from build123d import *

# Parameters (mm, degrees)
SKETCH2_R           = 6
BOSS_EXTRUDE1_DEPTH = 15
SKETCH3_R           = 6
CUT_EXTRUDE1_DEPTH  = 27
SKETCH4_R           = 6
CUT_EXTRUDE2_DEPTH  = 27


with BuildPart() as part:
    # Sketch2 → Boss-Extrude1 (new body)
    with BuildSketch(Plane.XY):
        Polygon((0, 20.4), (5, 25.4), (20.4, 25.4), (25.4, 20.4), (25.4, 5), (20.4, 0), (5, 0), (0, 5), align=None)
        with Locations((12.7, 12.7)):
            Circle(SKETCH2_R, mode=Mode.SUBTRACT)
    extrude(amount=BOSS_EXTRUDE1_DEPTH)

    # Sketch3 → Cut-Extrude1 (cut)
    with BuildSketch(Plane(origin=(25.4, 0, 0), x_dir=(0, 0, -1), z_dir=(1, 0, 0))):
        with Locations((-7.5, 12.7)):
            Circle(SKETCH3_R)
    extrude(amount=-CUT_EXTRUDE1_DEPTH, mode=Mode.SUBTRACT)

    # Sketch4 → Cut-Extrude2 (cut)
    with BuildSketch(Plane(origin=(0, 25.4, 0), x_dir=(1, 0, 0), z_dir=(0, 1, 0))):
        with Locations((12.7, -7.5)):
            Circle(SKETCH4_R)
    extrude(amount=-CUT_EXTRUDE2_DEPTH, mode=Mode.SUBTRACT)


solid = part.part
Work out the finished part from the listing and answer in its coordinate system (mm). Give positions to 0.01 mm unless a question says otherwise; leave off trailing zeros. Loops run counter-clockwise (first coordinate to the right, second up) from the corner with the lowest first, then second, coordinate; pieces in that order, holes last. Notation, with made-up numbers: (1.25, 42.5) -> (58.25, 42.5) arc R35 ccw to (58.25, 79.5) -> close; hole circle Ø1 at (48.25, 56). An arc over 180 degrees is marked (long way). Use a Markdown table: item, result. Add a question column.
1) The part is cut by section A-A, the plane x = 12.7. Determine the outline of the cut face in (y, z).
2) The part is cut by section C-C, the plane z = 9.5. Determine the outline of the cut face in (x, y), plus the area to 3 significant figures.
3) For a pull along X with two mould halves and no side action, classify faces 1 (the cylindrical face through (6.706, 12.964, 1.244)), 2 (the flat face through (9, 25.4, 2)), 3 (the flat face through (3, 2, 7)) as +X half, -X half, draft (parallel to the pull), parting line (faces both ways), or undercut.
4) Consider line 1 along Y through (x, z) = (12.7, 1); line 2 along Z through (x, y) = (12.75, 4.5); line 3 along Z through (x, y) = (3, 9). Determine where each line is inside the solid, lowest interval first.
5) The part is cut by section B-B, the plane y = 3. Determine the outline of the cut face in (x, z), plus the area to 3 significant figures.
6) This flat-tipped pin is pushed along its axis until it touches: P1, Ø11, axis at x = 12.7, y = 12.7, coming from the -Z side. Where does it stop, or does it pass through?
Reported:
| question | item | result |
|---|---|---|
| 1 | outline | (0, 0) -> (6.7, 0) -> (6.7, 1.5) -> (0, 1.5) -> close; (0, 13.5) -> (6.7, 13.5) -> (6.7, 15) -> (0, 15) -> close; (18.7, 0) -> (25.4, 0) -> (25.4, 1.5) -> (18.7, 1.5) -> close; (18.7, 13.5) -> (25.4, 13.5) -> (25.4, 15) -> (18.7, 15) -> close |
| 2 | outline | (0, 5) -> (5, 0) -> (7.04, 0) -> (7.04, 7.04) -> (0, 7.04) -> close; (0, 18.36) -> (7.04, 18.36) -> (7.04, 25.4) -> (5, 25.4) -> (0, 20.4) -> close; (18.36, 0) -> (20.4, 0) -> (25.4, 5) -> (25.4, 7.04) -> (18.36, 7.04) -> close; (18.36, 18.36) -> (25.4, 18.36) -> (25.4, 20.4) -> (20.4, 25.4) -> (18.36, 25.4) -> close |
| 2 | area | 148 mm^2 |
| 3 | face 1 | undercut |
| 3 | face 2 | draft |
| 3 | face 3 | -X half |
| 4 | line 1 | y = 0 to 6.7, 18.7 to 25.4 |
| 4 | line 2 | z = 0 to 1.5, 13.5 to 15 |
| 4 | line 3 | z = 0 to 2.78, 12.22 to 15 |
| 5 | outline | (2, 0) -> (23.4, 0) -> (23.4, 15) -> (2, 15) -> close; hole circle Ø12 at (12.7, 7.5) |
| 5 | area | 208 mm^2 |
| 6 | P1 | passes through |
